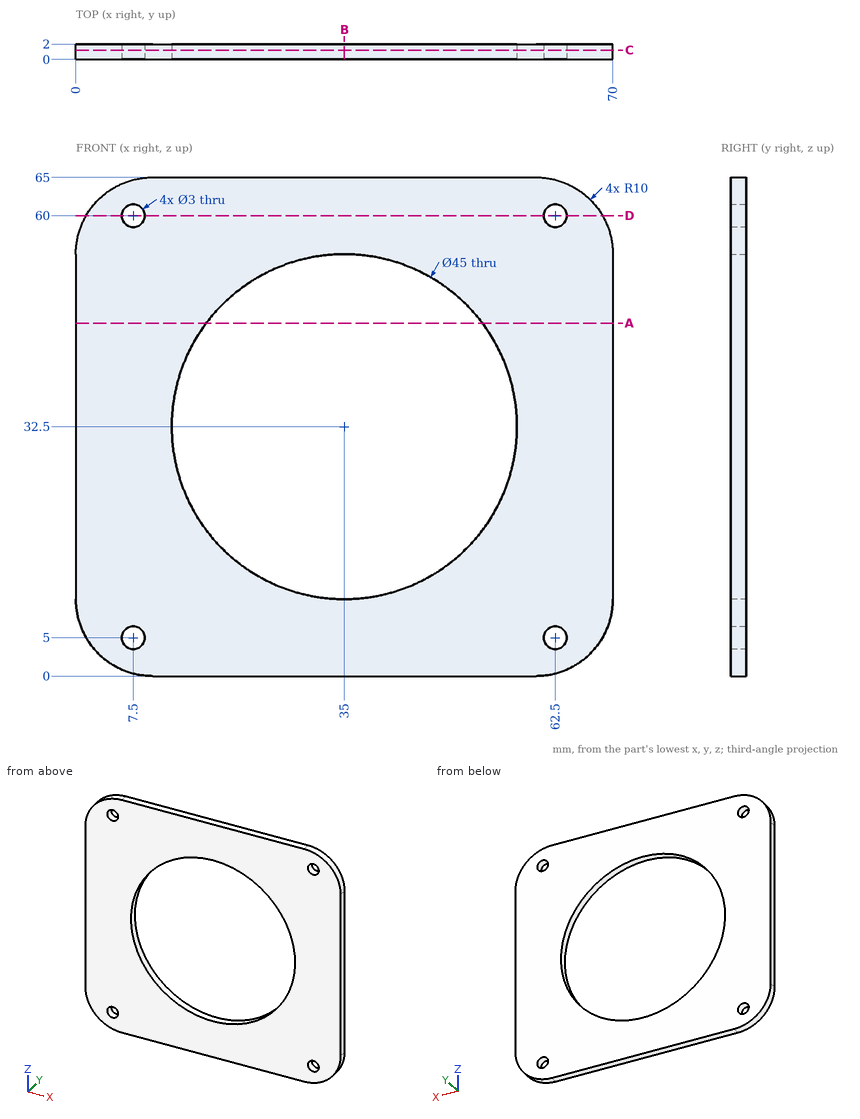
Verification items for this drawing (mm, ordinates from the low corner). Give positions to 0.01 mm unless a question says otherwise; leave off trailing zeros. Loops run counter-clockwise (first coordinate to the right, second up) from the corner with the lowest first, then second, coordinate; pieces in that order, holes last. Notation, with made-up numbers: M 8.5,73.25 L 64.5,73.25 A27 ccw 64.5,109.25 Z; hole C -7.75,58 d5. An arc over 180 degrees is marked long. Answer as a JSON object with one key per item and string values. Group by question number.
Q1. Cross-section at B-B on x = 35. Record the cut outline in (y, z), then the cut area to 3 significant figures.
Q2. Cross-section at A-A on z = 46. Record the cut outline in (x, y).
Q3. Go/stop test with flat-tipped pins: P1, Ø6, axis at x = 39, z = 16, coming from the +Y side; P2, Ø4, axis at x = 62.5, z = 5, coming from the -Y side. Record where each tip stops, or that it passes through.
Q4. Cross-section at C-C on y = 1.2. Record the cut outline in (x, z).
Q5. Cross-section at D-D on z = 60. Record the cut outline in (x, y), then the cut area to 3 significant figures.
Q6. Material ranges on line 1 along Z through (x, y) = (7.5, 1.05); line 2 along X through (y, z) = (1.3, 60); line 3 along X through (y, z) = (0.8, 41), recorded low to high. Write a range as [from, to].
Evaluation:
{
 "1": {"outline": "M 0,0 L 2,0 L 2,10 L 0,10 Z; M 0,55 L 2,55 L 2,65 L 0,65 Z", "area": "40.0 mm2"},
 "2": {"outline": "M 0,0 L 17,0 L 17,2 L 0,2 Z; M 53,0 L 70,0 L 70,2 L 53,2 Z"},
 "3": {"P1": "passes through", "P2": "stops at y = 0"},
 "4": {"outline": "M 0,10 A10 ccw 10,0 L 60,0 A10 ccw 70,10 L 70,55 A10 ccw 60,65 L 10,65 A10 ccw 0,55 Z; hole C 7.5,5 d3; hole C 7.5,60 d3; hole C 35,32.5 d45; hole C 62.5,5 d3; hole C 62.5,60 d3"},
 "5": {"outline": "M 1.34,0 L 6,0 L 6,2 L 1.34,2 Z; M 9,0 L 61,0 L 61,2 L 9,2 Z; M 64,0 L 68.66,0 L 68.66,2 L 64,2 Z", "area": "123 mm2"},
 "6": {"line 1": "z = [0.32, 3.5], [6.5, 58.5], [61.5, 64.68]", "line 2": "x = [1.34, 6], [9, 61], [64, 68.66]", "line 3": "x = [0, 14.17], [55.83, 70]"}
}
